from build123d import *

# Parameters (mm, degrees)
SKETCH1_W           = 1370
SKETCH1_H           = 900
BOSS_EXTRUDE1_DEPTH = 220
SHELL1_T            = -9
CUT_EXTRUDE1_REACH  = 1655.874
SKETCH3_W           = 615
SKETCH3_H           = 36


with BuildPart() as part:
    # Sketch1 → Boss-Extrude1 (new body)
    with BuildSketch(Plane(origin=(0, 0, 0), x_dir=(1, 0, 0), z_dir=(0, 1, 0))):
        with Locations((685, 450)):
            Rectangle(SKETCH1_W, SKETCH1_H)
    extrude(amount=BOSS_EXTRUDE1_DEPTH)

    # Shell1
    shell1_openings = [part.faces().sort_by_distance(p)[0] for p in [
        (685, 220, -450),
    ]]
    offset(amount=SHELL1_T, openings=shell1_openings, kind=Kind.INTERSECTION)

    # Sketch3 → Cut-Extrude1 (cut, up to next)
    with BuildSketch(Plane.XY, mode=Mode.PRIVATE) as cut_extrude1_sk1:
        with Locations((387.5, 168)):
            Rectangle(SKETCH3_W, SKETCH3_H)
    cut_extrude1_tool1 = extrude(cut_extrude1_sk1.sketch, amount=-CUT_EXTRUDE1_REACH, mode=Mode.PRIVATE) & part.part
    add(cut_extrude1_tool1.solids().sort_by_distance((387.5, 168, 0))[0], mode=Mode.SUBTRACT)


solid = part.part
Could you check a few things on this model? Use its own coordinates, in mm. A direction names the side the tool comes from. Give positions to 0.01 mm unless a question says otherwise; leave off trailing zeros. Order: outer loops, then holes, each group sorted by start corner. A loop starts at its lowest first (then second) coordinate and runs counter-clockwise, first axis right, second up.
Item 1: If we section it at B-B, the plane y = 56: Write out the boundary of the cut face in (x, z), plus the area to 3 significant figures.
Item 2: I need wall thicknesses on line 1 (X direction, y = 56.5, z = -534.5); line 2 (Z direction, x = 881, y = 29); line 3 (Y direction, x = 1026.5, z = -406). Which ranges of each line are inside material? Lowest first, please.
Item 3: If we section it at A-A, the plane x = 519: Write out the boundary of the cut face in (y, z).
Item 4: I'm going to push a flat-ended pin straight in: pin 1 (6 mm diameter, centred on x = 678.5, z = -699.5, fed in from +Y). Where does the tip first touch, or does it pass through?
Item 5: If we mould it in two halves opening along Z, with no side actions, what happens to faces 1 (the face through (0, 108, -444)), 2 (the face through (675, 108, -900)), 3 (the face through (1361, 113, -444)), 4 (the face through (676, 9, -456))? For each: pulls with the +Z half, pulls with the -Z half, needs draft (parallel to the pull), parting line crosses it, or undercut.
Item 6: If we section it at D-D, the plane x = 891.5: Write out the boundary of the cut face in (y, z), plus the area to 3 significant figures.
Item 7: For faces 5 (the face through (676, 113, -9)), 6 (the face through (675, 0, -456)), which set-ups out of +Z, -Z, +X, -X, +Y, -Y let a thin tool reach every point of the face, with its end or its side?
Item 8: If we section it at C-C, the plane z = -160: Write out the boundary of the cut face in (x, y), plus the area to 3 significant figures.
Values:
1. outline: (0, -900) - (1370, -900) - (1370, 0) - (0, 0) - close; hole (9, -891) - (1361, -891) - (1361, -9) - (9, -9) - close
1. area: 40,500 mm2
2. line 1: x = 0 to 9, 1361 to 1370
2. line 2: z = -900 to -891, -9 to 0
2. line 3: y = 0 to 9
3. outline: (0, -900) - (220, -900) - (220, -891) - (9, -891) - (9, -9) - (150, -9) - (150, 0) - (0, 0) - close; (186, -9) - (220, -9) - (220, 0) - (186, 0) - close
4. pin 1: stops at y = 9
5. face 1: needs draft
5. face 2: pulls with the -Z half
5. face 3: undercut
5. face 4: undercut
6. outline: (0, -900) - (220, -900) - (220, -891) - (9, -891) - (9, -9) - (220, -9) - (220, 0) - (0, 0) - close
6. area: 11,900 mm2
7. face 5: +Y
7. face 6: +Z, -Z, +X, -X, -Y
8. outline: (0, 0) - (1370, 0) - (1370, 220) - (1361, 220) - (1361, 9) - (9, 9) - (9, 220) - (0, 220) - close
8. area: 16,100 mm2
